from build123d import *

# Parameters (mm, degrees)
F0_R     = 7.5
F0_R_2   = 12.5
F1_DEPTH = 7
F3_D     = 5
F4_SIZE  = 0.5


with BuildPart() as f1:
    # F0 (on Front) → F1 (new body)
    with BuildSketch(Plane.XZ):
        with BuildLine():
            ThreePointArc((-53.3733215365, -4.6372554806), (-53.6928232219, -22.8167624061), (-38, -32))
            Line((-38, -32), (38, -32))
            ThreePointArc((38, -32), (53.6928232219, -22.8167624061), (53.3733215365, -4.6372554806))
            Line((53.3733215365, -4.6372554806), (15.3733215365, 57.7575067788))
            ThreePointArc((15.3733215365, 57.7575067788), (0, 66.3947622594), (-15.3733215365, 57.7575067788))
            Line((-15.3733215365, 57.7575067788), (-53.3733215365, -4.6372554806))
        make_face()
        with Locations((-38, -14)):
            Circle(F0_R, mode=Mode.SUBTRACT)
        with Locations((38, -14)):
            Circle(F0_R, mode=Mode.SUBTRACT)
        Circle(F0_R_2, mode=Mode.SUBTRACT)
        with Locations((0, 48.3947622594)):
            Circle(F0_R, mode=Mode.SUBTRACT)
    extrude(amount=F1_DEPTH)

    # F3 (through all)
    with Locations(Plane.XZ.offset(7)):
        with Locations((-15.1554445662, 8.75), (15.1554445662, 8.75), (0, -17.5)):
            Hole(F3_D / 2)

    # F4
    f4_edges = [f1.edges().sort_by_distance(p)[0] for p in [
        (-53.692823, -7, -22.816762),
        (-34.373322, -7, 26.560126),
        (0, -7, -32),
        (0, -7, 66.394762),
        (53.692823, -7, -22.816762),
        (34.373322, -7, 26.560126),
        (-45.5, -7, -14),
        (-17.655445, -7, 8.75),
        (-2.5, -7, -17.5),
        (30.5, -7, -14),
        (-12.5, -7, 0),
        (12.655445, -7, 8.75),
        (-7.5, -7, 48.394762),
        (-53.692823, 0, -22.816762),
        (-34.373322, 0, 26.560126),
        (0, 0, -32),
        (0, 0, 66.394762),
        (53.692823, 0, -22.816762),
        (34.373322, 0, 26.560126),
        (-45.5, 0, -14),
        (-17.655445, 0, 8.75),
        (-2.5, 0, -17.5),
        (30.5, 0, -14),
        (-12.5, 0, 0),
        (12.655445, 0, 8.75),
        (-7.5, 0, 48.394762),
    ]]
    chamfer(f4_edges, length=F4_SIZE)


solid = f1.part
The model under review builds one solid part; all positions refer to its coordinate system, in mm. Give positions to 0.01 mm unless a question says otherwise; leave off trailing zeros. Loops run counter-clockwise (first coordinate to the right, second up) from the corner with the lowest first, then second, coordinate; pieces in that order, holes last. Notation, with made-up numbers: (-25, 51.25) -> (7, 51.25) arc R24 ccw to (7, 62.25) -> close; hole circle Ø9 at (7, -7.75). An arc over 180 degrees is marked (long way). Answer as a JSON object with one key per item and string values. Group by question number.
Q1. Wall thickness on line 1 along X through (y, z) = (-6, 6.5); line 2 along X through (y, z) = (-0.5, -9.5); line 3 along Z through (x, y) = (-8.5, -2.75): over which ranges is each line inside the solid? List them lowest first.
Q2. Insertion check: pin 1 (1.5 mm diameter, centred on x = 42.5, y = -5, fed in from +Z); pin 2 (3 mm diameter, centred on y = -5.5, z = -13, fed in from +X); pin 3 (4 mm diameter, centred on y = -2.5, z = 27, fed in from -X); pin 4 (4 mm diameter, centred on y = -2.5, z = 26.5, fed in from +X). Each pin has a flat end and moves straight along its axis. Give the tip position at first contact, or say it passes through.
Q3. Take a section at B-B (y = -3). Write out the cut boundary in (x, z), plus the area to 3 significant figures.
Q4. Draft analysis for pull direction Z (two halves, no side actions). For faces 1 (the cylindrical face through (-13.17, -3.46, 7.23)), 2 (the conical face through (53.25, -0.14, -22.87)), 3 (the flat face through (-34.107, -3.458, 26.997)), state which applies: pulls with the +Z half, pulls with the -Z half, needs draft (parallel to the pull), parting line crosses it, or undercut.
Q5. Take a section at A-A (x = 0). State how many separate pieces and enclosed holes the cut face has, plus the area to 3 significant figures.
Q6. Take a section at C-C (z = 36.5). Write out the cut boundary in (x, y).
Answer below:
{
 "1": {"line 1": "x = -46.59 to -16.25, -14.07 to -10.68, 10.68 to 14.07, 16.25 to 46.59", "line 2": "x = -55.43 to -44, -32 to -8.12, 8.12 to 32, 44 to 55.43", "line 3": "z = -32 to -9.17, 9.17 to 64.26"},
 "2": {"pin 1": "stops at z = 14.45", "pin 2": "stops at x = 56", "pin 3": "stops at x = -35.32", "pin 4": "stops at x = 35.63"},
 "3": {"outline": "(-53.37, -4.64) arc R18 ccw to (-38, -32) -> (38, -32) arc R18 ccw to (53.37, -4.64) -> (15.37, 57.76) arc R18 ccw to (-15.37, 57.76) -> close; hole circle Ø15 at (-38, -14); hole circle Ø5 at (-15.16, 8.75); hole circle Ø25 at (0, 0); hole circle Ø15 at (0, 48.39); hole circle Ø5 at (0, -17.5); hole circle Ø5 at (15.16, 8.75); hole circle Ø15 at (38, -14)", "area": "6,310 mm2"},
 "4": {"face 1": "undercut", "face 2": "parting line crosses it", "face 3": "pulls with the +Z half"},
 "5": {"separate pieces": "4", "enclosed holes": "0", "area": "372 mm2"},
 "6": {"outline": "(-28.32, -6.5) -> (-27.73, -7) -> (27.73, -7) -> (28.32, -6.5) -> (28.32, -0.5) -> (27.73, 0) -> (-27.73, 0) -> (-28.32, -0.5) -> close"}
}
